Verification items for the finished model (mm, model axes). Face numbers are marked on the shaded views. A direction names the side the tool comes from. Give positions to 0.01 mm unless a question says otherwise; leave off trailing zeros. Loops run counter-clockwise (first coordinate to the right, second up) from the corner with the lowest first, then second, coordinate; pieces in that order, holes last. Notation, with made-up numbers: M 75.5,79.5 L 121.5,79.5 A9 ccw 121.5,86.5 Z; hole C 44.25,-35 d7. An arc over 180 degrees is marked long. Use CSV: the item, a comma, the result in double quotes.
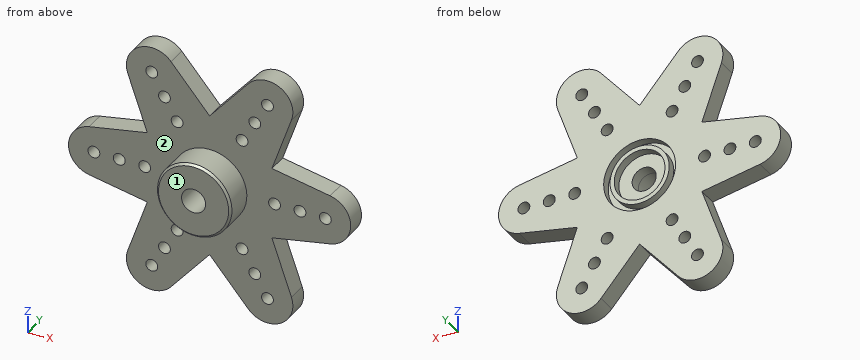
from build123d import *

# Parameters (mm, degrees)
SKETCH_1_R          = 0.7
EXTRUDE_1_DEPTH     = 2.35
SKETCH_2_R          = 4.4
SKETCH_2_R_2        = 1.425
EXTRUDE_2_DEPTH     = 3.5
SKETCH_3_R          = 1.425
CUT_EXTRUDE_1_DEPTH = 23.59684111
SKETCH_4_R          = 3
SKETCH_4_R_2        = 1.425
CUT_EXTRUDE_2_DEPTH = 1
SKETCH_4_3_R        = 4.25
SKETCH_4_3_R_2      = 3.5
CUT_EXTRUDE_3_DEPTH = 1
CHAMFER_1_SIZE      = 0.25


with BuildPart() as part:
    # Sketch 1 → Extrude 1 (new body)
    with BuildSketch(Plane(origin=(0, 0, 0), x_dir=(1, 0, 0), z_dir=(0, 1, 0))):
        with BuildLine():
            Line((-7.361215932, -4.25), (-14.233620573, -2.947531689))
            ThreePointArc((-14.233620573, -2.947531689), (-16.675, 0), (-14.233620573, 2.947531689))
            Line((-14.233620573, 2.947531689), (-7.361215932, 4.25))
            Line((-7.361215932, 4.25), (-9.669447607, 10.85291116))
            ThreePointArc((-9.669447607, 10.85291116), (-8.3375, 14.440973608), (-4.564172966, 13.800442848))
            Line((-4.564172966, 13.800442848), (0, 8.499999999))
            Line((0, 8.499999999), (4.564172966, 13.800442848))
            ThreePointArc((4.564172966, 13.800442848), (8.3375, 14.440973608), (9.669447607, 10.852911159))
            Line((9.669447607, 10.852911159), (7.361215932, 4.25))
            Line((7.361215932, 4.25), (14.233620573, 2.947531688))
            ThreePointArc((14.233620573, 2.947531688), (16.675, -1e-09), (14.233620573, -2.947531689))
            Line((14.233620573, -2.947531689), (7.361215932, -4.25))
            Line((7.361215932, -4.25), (9.669447607, -10.852911161))
            ThreePointArc((9.669447607, -10.852911161), (8.337499999, -14.440973608), (4.564172965, -13.800442849))
            Line((4.564172965, -13.800442849), (0, -8.5))
            Line((0, -8.5), (-4.564172966, -13.800442849))
            ThreePointArc((-4.564172966, -13.800442849), (-8.3375, -14.440973608), (-9.669447608, -10.85291116))
            Line((-9.669447608, -10.85291116), (-7.361215932, -4.25))
        make_face()
        with Locations(Location((-13.675, 0, 0), (0, 0, 270))):
            Circle(SKETCH_1_R, mode=Mode.SUBTRACT)
        with Locations(Location((-10.675, 0, 0), (0, 0, 270))):
            Circle(SKETCH_1_R, mode=Mode.SUBTRACT)
        with Locations(Location((-7.675, 0, 0), (0, 0, 270))):
            Circle(SKETCH_1_R, mode=Mode.SUBTRACT)
        with Locations(Location((-6.8375, 11.842897397, 0), (0, 0, 270))):
            Circle(SKETCH_1_R, mode=Mode.SUBTRACT)
        with Locations(Location((-5.3375, 9.244821185, 0), (0, 0, 270))):
            Circle(SKETCH_1_R, mode=Mode.SUBTRACT)
        with Locations(Location((-3.8375, 6.646744974, 0), (0, 0, 270))):
            Circle(SKETCH_1_R, mode=Mode.SUBTRACT)
        with Locations(Location((6.8375, 11.842897397, 0), (0, 0, 270))):
            Circle(SKETCH_1_R, mode=Mode.SUBTRACT)
        with Locations(Location((5.3375, 9.244821185, 0), (0, 0, 270))):
            Circle(SKETCH_1_R, mode=Mode.SUBTRACT)
        with Locations(Location((3.8375, 6.646744974, 0), (0, 0, 270))):
            Circle(SKETCH_1_R, mode=Mode.SUBTRACT)
        with Locations(Location((13.675, 0, 0), (0, 0, 270))):
            Circle(SKETCH_1_R, mode=Mode.SUBTRACT)
        with Locations(Location((10.675, 0, 0), (0, 0, 270))):
            Circle(SKETCH_1_R, mode=Mode.SUBTRACT)
        with Locations(Location((7.675, 0, 0), (0, 0, 270))):
            Circle(SKETCH_1_R, mode=Mode.SUBTRACT)
        with Locations(Location((6.8375, -11.842897397, 0), (0, 0, 270))):
            Circle(SKETCH_1_R, mode=Mode.SUBTRACT)
        with Locations(Location((5.3375, -9.244821185, 0), (0, 0, 270))):
            Circle(SKETCH_1_R, mode=Mode.SUBTRACT)
        with Locations(Location((3.8375, -6.646744974, 0), (0, 0, 270))):
            Circle(SKETCH_1_R, mode=Mode.SUBTRACT)
        with Locations(Location((-6.8375, -11.842897397, 0), (0, 0, 270))):
            Circle(SKETCH_1_R, mode=Mode.SUBTRACT)
        with Locations(Location((-5.3375, -9.244821185, 0), (0, 0, 270))):
            Circle(SKETCH_1_R, mode=Mode.SUBTRACT)
        with Locations(Location((-3.8375, -6.646744974, 0), (0, 0, 270))):
            Circle(SKETCH_1_R, mode=Mode.SUBTRACT)
    extrude(amount=EXTRUDE_1_DEPTH)

    # Sketch 2 → Extrude 2 (add)
    with BuildSketch(Plane.XZ):
        with Locations(Location((0, 0, 0), (0, 0, 90))):
            Circle(SKETCH_2_R)
        with Locations(Location((0, 0, 0), (0, 0, 270))):
            Circle(SKETCH_2_R_2, mode=Mode.SUBTRACT)
    extrude(amount=EXTRUDE_2_DEPTH)

    # Sketch 3 → Cut-Extrude 1 (cut, through all)
    with BuildSketch(Plane.XZ):
        with Locations(Location((0, 0, 0), (0, 0, 270))):
            Circle(SKETCH_3_R)
    extrude(amount=-CUT_EXTRUDE_1_DEPTH, mode=Mode.SUBTRACT)

    # Sketch 4 → Cut-Extrude 2 (cut)
    with BuildSketch(Plane(origin=(0, 2.35, 0), x_dir=(1, 0, 0), z_dir=(0, 1, 0))):
        with Locations(Location((0, 0, 0), (0, 0, 270))):
            Circle(SKETCH_4_R)
        with Locations(Location((0, 0, 0), (0, 0, 270))):
            Circle(SKETCH_4_R_2, mode=Mode.SUBTRACT)
    extrude(amount=-CUT_EXTRUDE_2_DEPTH, mode=Mode.SUBTRACT)

    # Sketch 4_3 → Cut-Extrude 3 (cut)
    with BuildSketch(Plane(origin=(0, 2.35, 0), x_dir=(1, 0, 0), z_dir=(0, 1, 0))):
        with Locations(Location((0, 0, 0), (0, 0, 270))):
            Circle(SKETCH_4_3_R)
        with Locations(Location((0, 0, 0), (0, 0, 270))):
            Circle(SKETCH_4_3_R_2, mode=Mode.SUBTRACT)
    extrude(amount=-CUT_EXTRUDE_3_DEPTH, mode=Mode.SUBTRACT)

    # Chamfer 1
    chamfer_1_edges = [part.edges().sort_by_distance(p)[0] for p in [
        (0, -3.5, -4.4),
    ]]
    chamfer(chamfer_1_edges, length=CHAMFER_1_SIZE)


solid = part.part
(1) Section check B-B on z = 9.25. Record the cut outline in (x, y).
Calculated:
outline,"M -9.11,0 L -6.04,0 L -6.04,2.35 L -9.11,2.35 Z; M -4.64,0 L -0.65,0 L -0.65,2.35 L -4.64,2.35 Z; M 0.65,0 L 4.64,0 L 4.64,2.35 L 0.65,2.35 Z; M 6.04,0 L 9.11,0 L 9.11,2.35 L 6.04,2.35 Z"
(2) Tool access check on the marked faces 1 and 2. Record the directions out of +Z, -Z, +X, -X, +Y, -Y that give a thin tool (end or side, any length) a straight path to the whole face; none if there is none.
Calculated:
face 1,"+Z, -Z, +X, -X, -Y"
face 2,"-Y"
(3) Section check D-D on z = 5.5. Record the cut outline in (x, y).
Calculated:
outline,"M -7.8,0 L 7.8,0 L 7.8,2.35 L -7.8,2.35 Z"
(4) Section check C-C on y = -1.3. Record the cut outline in (x, z) (3 decimals).
Calculated:
outline,"C 0,0 d8.8; hole C 0,0 d2.85"
(5) Scan lines: L1, parallel to X at y = 0.9, z = -11.5; L2, parallel to X at y = 0.7, z = 7; L3, parallel to Y at x = 8, z = 1.25. Record each from-to range of solid material in increasing order. Write a range as from..to.
Calculated:
L1,"x = -9.82..-7.45, -6.23..-2.58, 2.58..6.23, 7.45..9.82"
L2,"x = -8.32..-4.44, -3.23..3.23, 4.44..8.32"
L3,"y = 0..2.35"
(6) Section check A-A on z = 0. Count the separate pieces of the cut face and the enclosed holes in it, plus the area to 3 significant figures.
Calculated:
separate pieces,"8"
enclosed holes,"0"
area,"68.0 mm²"
(7) Depth check by flat-ended pin: pin 1 Ø5 at (x, z) = (8.5, -6) entering from -Y; pin 2 Ø1 at (y, z) = (1.5, -1) entering from +X. Enter the tip coordinate at first touch or a pass-through.
Calculated:
pin 1,"stops at y = 0"
pin 2,"stops at x = 16.63"
